Can you work these out from the model? Positions are in its coordinate system, mm. Round coordinates to 2 decimals unless told otherwise and drop trailing zeros. Loops run counter-clockwise (first coordinate to the right, second up) from the corner with the lowest first, then second, coordinate; pieces in that order, holes last. Notation, with made-up numbers: (42, 27) - (65, 27) arc R23 ccw to (65, 41) - close; hole circle Ø3 at (-32, 34.5). An arc over 180 degrees is marked (long way). Answer as CSV lines item,"result".
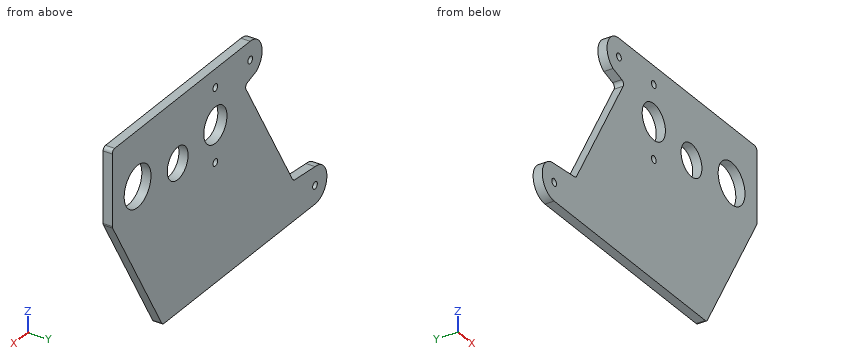
```python
from build123d import *

# Parameters (mm, degrees)
SKETCH1_R           = 2.4892
SKETCH1_R_2         = 14.3002
SKETCH1_R_3         = 11.1252
SKETCH1_R_4         = 12.3825
BOSS_EXTRUDE1_DEPTH = 6.35
CUT_EXTRUDE3_DEPTH  = 196.570791382
FILLET2_R           = 2.54


with BuildPart() as part:
    # Sketch1 → Boss-Extrude1 (new body)
    with BuildSketch(Plane(origin=(0, 0, 0), x_dir=(1, 0, 0), z_dir=(0, 1, 0))):
        with BuildLine():
            ThreePointArc((-168.788743889, 72.590962133), (-181.488743889, 59.890962122), (-168.788743866, 47.190962133))
            Line((-168.788743866, 47.190962133), (-145.58139547, 45.094655563))
            Line((-145.58139547, 45.094655563), (-93.510572414, -45.094655563))
            Line((-93.510572414, -45.094655563), (-105.98261767, -48.892439505))
            ThreePointArc((-105.98261767, -48.892439505), (-111.899875664, -63.177964006), (-99.63261767, -72.590962133))
            Line((-99.63261767, -72.590962133), (47.56445351, -72.590962133))
            Line((47.56445351, -72.590962133), (47.56445351, 72.590962133))
            Line((47.56445351, 72.590962133), (-168.788743889, 72.590962133))
        make_face()
        with Locations(Location((-168.788743889, 59.890962133, 0), (0, 0, 270))):
            Circle(SKETCH1_R, mode=Mode.SUBTRACT)
        with Locations(Location((20.56425351, -34.490962133, 0), (0, 0, 270))):
            Circle(SKETCH1_R_2, mode=Mode.SUBTRACT)
        with Locations(Location((-22.22178223, -28.671379192, 0), (0, 0, 270))):
            Circle(SKETCH1_R_3, mode=Mode.SUBTRACT)
        with Locations(Location((-62.44294649, -9.090962133, 0), (0, 0, 270))):
            Circle(SKETCH1_R, mode=Mode.SUBTRACT)
        with Locations(Location((-62.44294649, -34.490962133, 0), (0, 0, 270))):
            Circle(SKETCH1_R_4, mode=Mode.SUBTRACT)
        with Locations(Location((-62.44294649, -59.890962133, 0), (0, 0, 270))):
            Circle(SKETCH1_R, mode=Mode.SUBTRACT)
        with Locations(Location((-99.63261767, -59.890962133, 0), (0, 0, 270))):
            Circle(SKETCH1_R, mode=Mode.SUBTRACT)
    extrude(amount=BOSS_EXTRUDE1_DEPTH)

    # Sketch3 → Cut-Extrude3 (cut, through all)
    with BuildSketch(Plane(origin=(0, 6.35, 0), x_dir=(1, 0, 0), z_dir=(0, 1, 0))):
        Polygon((47.56445351, -20.190762133), (-6.003099971, 72.590962133), (47.56445351, 72.590962133), align=None)
    extrude(amount=-CUT_EXTRUDE3_DEPTH, mode=Mode.SUBTRACT)

    # Fillet2
    fillet2_edges = [part.edges().sort_by_distance(p)[0] for p in [
        (-93.510572414, 3.175, 45.094655563),
        (-145.58139547, 3.175, -45.094655563),
        (47.56445351, 3.175, 72.590962133),
        (47.56445351, 3.175, 20.190762133),
        (-6.003099971, 3.175, -72.590962133),
    ]]
    fillet(fillet2_edges, radius=FILLET2_R)


solid = part.part
```
Q1. Imagine slicing it at B-B (y = 1.5). Write out the boundary of the cut face in (x, z) (1 decimal), then the cut area to 3 significant figures.
Checks:
outline,"(-168.8, -72.6) - (-7.5, -72.6) arc R2.5 ccw to (-5.3, -71.3) - (47.2, 19.6) arc R2.5 ccw to (47.6, 20.9) - (47.6, 70.1) arc R2.5 ccw to (45, 72.6) - (-99.6, 72.6) arc R12.7 ccw to (-106, 48.9) - (-96.6, 46) arc R2.5 cw to (-95.1, 42.3) - (-144.9, -44) arc R2.5 cw to (-146.9, -45.2) - (-168.8, -47.2) arc R12.7 ccw to start; hole circle Ø5 at (-168.8, -59.9); hole circle Ø5 at (-99.6, 59.9); hole circle Ø24.8 at (-62.4, 34.5); hole circle Ø5 at (-62.4, 9.1); hole circle Ø5 at (-62.4, 59.9); hole circle Ø22.3 at (-22.2, 28.7); hole circle Ø28.6 at (20.6, 34.5)"
area,"21,500 mm²"
Q2. Imagine slicing it at C-C (z = -31). Write out the boundary of the cut face in (x, y).
Checks:
outline,"(-137.44, 0) - (18.01, 0) - (18.01, 6.35) - (-137.44, 6.35) - close"
Q3. Imagine slicing it at D-D (x = 16). Write out the boundary of the cut face in (y, z).
Checks:
outline,"(0, -34.48) - (6.35, -34.48) - (6.35, 20.94) - (0, 20.94) - close; (0, 48.04) - (6.35, 48.04) - (6.35, 72.59) - (0, 72.59) - close"
Q4. I'm going to push a flat-ended pin straight in: pin 1 Ø3 at (y, z) = (3, -54) entering from +X. Where does the tip first touch, or does it pass through?
Checks:
pin 1,"x = 5.6"
Q5. Imagine slicing it at A-A (x = -55). Write out the boundary of the cut face in (y, z).
Checks:
outline,"(0, -72.59) - (6.35, -72.59) - (6.35, 24.6) - (0, 24.6) - close; (0, 44.39) - (6.35, 44.39) - (6.35, 72.59) - (0, 72.59) - close"
Q6. If I drill on line 1 along X through (y, z) = (4, 59.5); line 2 along X through (y, z) = (4.5, 45); line 3 along X through (y, z) = (3.25, -61), over which ranges is the centre line in solid material (lowest first)? Write a range as [from, to].
Checks:
line 1,"[-112.33, -102.09], [-97.17, -64.9], [-59.98, 47.56]"
line 2,"[-95.19, -68.99], [-55.89, 10.87], [30.26, 47.56]"
line 3,"[-181.44, -171.02], [-166.56, 0.69]"
